Study the drawing (mm; zero at the part's minimum x, y, z) and answer. A direction names the side the tool comes from. Coordinates: 2 decimals unless noted, no trailing zeros. Loops run counter-clockwise (first coordinate to the right, second up) from the corner with the lowest first, then second, coordinate; pieces in that order, holes last. Notation, with made-up numbers: (8, 57.25) - (30, 57.25) arc R13 cw to (30, 76.25) - close; hole circle Ø10 at (81, 7.5). An arc over 180 degrees is marked (long way). Use one line per item in the form item = value.
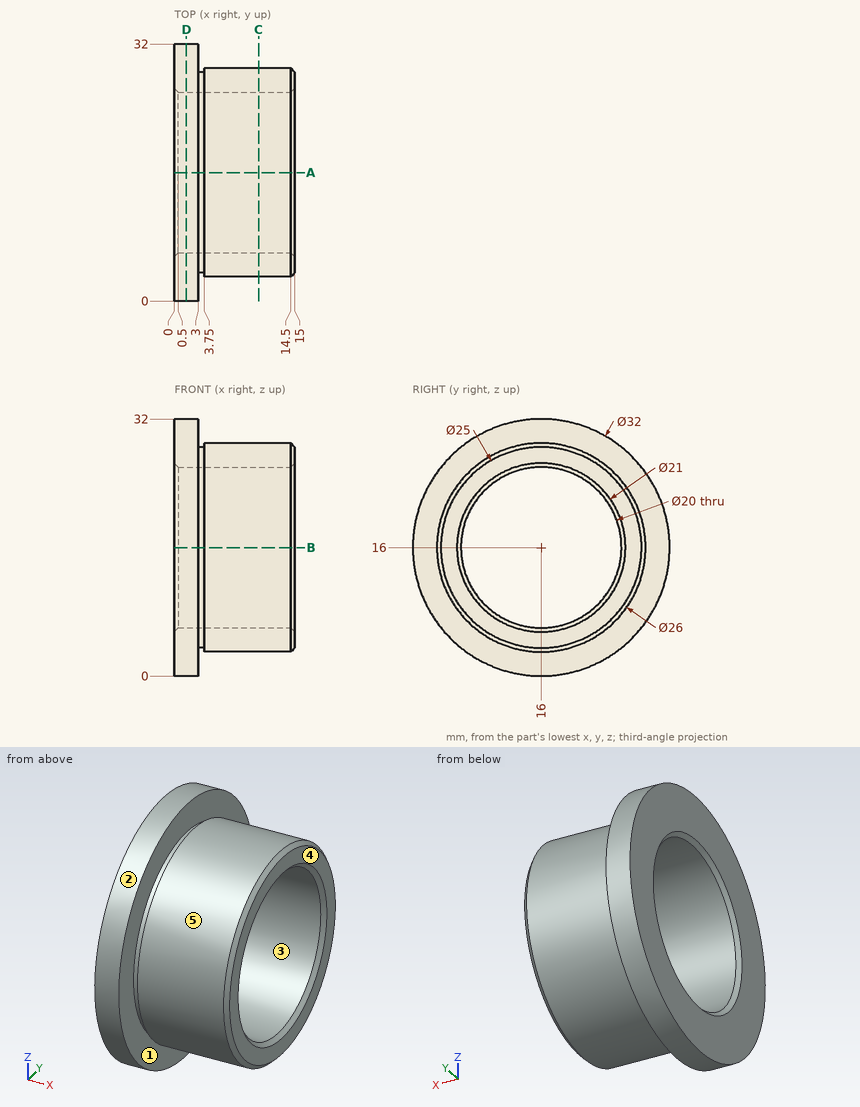
Item 1: Which of the six approach directions +Z, -Z, +X, -X, +Y, -Y give full straight-line access (tool end or side, diameter ignored) to the marked faces 4 and 5?
Results below:
face_4 = +Z, -Z, +X, +Y, -Y
face_5 = +X
Item 2: The part is cut by section A-A on y = 16. Give the vertices of the cut face in (x, z).
Results below:
outline = (0, 0) - (3, 0) - (3, 3.5) - (3.75, 3.5) - (3.75, 3) - (14.5, 3) - (15, 3.5) - (15, 5.5) - (14.5, 6) - (0.5, 6) - (0, 5.5) - close; (0, 26.5) - (0.5, 26) - (14.5, 26) - (15, 26.5) - (15, 28.5) - (14.5, 29) - (3.75, 29) - (3.75, 28.5) - (3, 28.5) - (3, 32) - (0, 32) - close
Item 3: Find the intervals of material crossed by L1, parallel to Y at x = 9.25, z = 16; L2, parallel to X at y = 26.5, z = 7, in increasing order.
Results below:
L1 = 3 to 6, 26 to 29
L2 = 0 to 3
Item 4: Each of these flat-tipped pins is pushed along its axis until it touches: P1, Ø9.5, axis at y = 12.5, z = 11.5, coming from the +X side; P2, Ø4, axis at y = 9, z = 14.5, coming from the +X side; P3, Ø1.5, axis at x = 4.5, y = 7.5, coming from the +Z side; P4, Ø8, axis at x = 10.5, y = 16.5, coming from the -Z side. Where does it stop, or does it pass through?
Results below:
P1 = 14.95
P2 = through
P3 = 26.44
P4 = 3
Item 5: For a pull along Y with two mould halves and no side action, classify the marked faces 1, 2 and 3 as +Y half, -Y half, draft (parallel to the pull), parting line (faces both ways), or undercut.
Results below:
face_1 = draft
face_2 = parting line
face_3 = undercut
Item 6: The part is cut by section D-D on x = 1.5. Give the vertices of the cut face in (y, z).
Results below:
outline = circle Ø32 at (16, 16); hole circle Ø20 at (16, 16)
Item 7: The part is cut by section C-C on x = 10.5. Give the vertices of the cut face in (y, z), plus the area to 3 significant figures.
Results below:
outline = circle Ø26 at (16, 16); hole circle Ø20 at (16, 16)
area = 217 mm²
